```python
from build123d import *

# Parameters (mm, degrees)
SKETCH1_W                                           = 128
SKETCH1_H                                           = 28
BOSS_EXTRUDE1_DEPTH                                 = 45
SKETCH2_OUTSIDE_W                                   = 157.708
SKETCH2_OUTSIDE_H                                   = 74.708
CUT_EXTRUDE2_DEPTH                                  = 84.096329642
FILLET1_R                                           = 6
FILLET2_R                                           = 2
SKETCH3_W                                           = 16
SKETCH3_H                                           = 16
CUT_EXTRUDE3_DEPTH                                  = 29
FILLET3_R                                           = 2
CBORE_FOR_M8_HEX_SOCKET_HEAD_CAP_SCREW1_D           = 9
CBORE_FOR_M8_HEX_SOCKET_HEAD_CAP_SCREW1_DEPTH       = 15
CBORE_FOR_M8_HEX_SOCKET_HEAD_CAP_SCREW1_CBORE_D     = 15
CBORE_FOR_M8_HEX_SOCKET_HEAD_CAP_SCREW1_CBORE_DEPTH = 8.6
CBORE_FOR_M8_HEX_SOCKET_HEAD_CAP_SCREW1_TIP         = 2.703872786


with BuildPart() as part:
    # Sketch1 → Boss-Extrude1 (new body)
    with BuildSketch(Plane.XY):
        Rectangle(SKETCH1_W, SKETCH1_H)
    extrude(amount=BOSS_EXTRUDE1_DEPTH)

    # Sketch2 outside → Cut-Extrude2 (cut, through all)
    with BuildSketch(Plane.XZ.offset(14)):
        with Locations((0, 22.5)):
            Rectangle(SKETCH2_OUTSIDE_W, SKETCH2_OUTSIDE_H)
        Polygon((-47, 0), (-47, 38), (47, 38), (47, 0), (64, 0), (64, 16), (51, 45), (-51, 45), (-64, 16), (-64, 0), align=None, mode=Mode.SUBTRACT)
    extrude(amount=-CUT_EXTRUDE2_DEPTH, mode=Mode.SUBTRACT)

    # Fillet1
    fillet1_edges = [part.edges().sort_by_distance(p)[0] for p in [
        (-64, 0, 16),
        (-51, 0, 45),
        (51, 0, 45),
        (64, 0, 16),
    ]]
    fillet(fillet1_edges, radius=FILLET1_R)

    # Fillet2
    fillet2_edges = [part.edges().sort_by_distance(p)[0] for p in [
        (-47, 14, 19),
        (0, 14, 38),
        (47, -14, 19),
        (47, 14, 19),
        (47, 0, 38),
        (0, -14, 38),
        (-47, 0, 38),
        (-47, -14, 19),
        (0, -14, 45),
        (0, 14, 45),
        (-58.032245896, -14, 29.312682233),
        (-64, -14, 7.358346808),
        (64, -14, 7.358346808),
        (58.032245896, -14, 29.312682233),
        (63.867296468, -14, 15.971616785),
        (50.375820334, -14, 44.036169802),
        (-63.867296468, -14, 15.971616785),
        (-50.375820334, -14, 44.036169802),
        (-58.032245896, 14, 29.312682233),
        (58.032245896, 14, 29.312682233),
        (64, 14, 7.358346808),
        (-64, 14, 7.358346808),
        (63.867296468, 14, 15.971616785),
        (50.375820334, 14, 44.036169802),
        (-63.867296468, 14, 15.971616785),
        (-50.375820334, 14, 44.036169802),
    ]]
    fillet(fillet2_edges, radius=FILLET2_R)

    # Sketch3 → Cut-Extrude3 (cut)
    with BuildSketch(Plane.XY.offset(45)):
        with Locations((-56, 0)):
            Rectangle(SKETCH3_W, SKETCH3_H)
        with Locations((56, 0)):
            Rectangle(SKETCH3_W, SKETCH3_H)
    extrude(amount=-CUT_EXTRUDE3_DEPTH, mode=Mode.SUBTRACT)

    # Fillet3
    # the kernel refuses this fillet: 2 mm, written as the material it takes off along each edge
    with BuildSketch(Plane(origin=(63.861153873, -8, 16), x_dir=(0.06925637128898768, 0, -0.9975988948650063), z_dir=(0, 1, 0))) as fillet3_piece_1:
        with BuildLine():
            CenterArc((1.866301026, 1.99519779), FILLET3_R, 183.971276773, 90)
            Line((-0.128896764, 1.856685047), (-0.328416543, 1.842833773))
            Line((-0.328416543, 1.842833773), (-0.199519779, -0.013851274))
            Line((-0.199519779, -0.013851274), (-0.029143426, -0.197865259))
            ThreePointArc((-0.029143426, -0.197865259), (1.303692283, -0.249155378), (2.018665043, -0.199519779))
            Line((2.018665043, -0.199519779), (2.004813769, 0))
        make_face()
    extrude(amount=16, mode=Mode.SUBTRACT)
    with BuildSketch(Plane(origin=(48, -8, 44.934279824), x_dir=(-0.999460544146637, 0, 0.032842361274859504), z_dir=(0, 1, 0))) as fillet3_piece_2:
        with BuildLine():
            CenterArc((1.935394771, -1.998921088), FILLET3_R, 88.117932867, 90)
            Line((-0.063526317, -1.933236366), (-0.263418426, -1.926667893))
            Line((-0.263418426, -1.926667893), (-0.199892109, 0.006568472))
            Line((-0.199892109, 0.006568472), (-0.02300822, 0.198672147))
            ThreePointArc((-0.02300822, 0.198672147), (0.893869228, 0.236490976), (2.007647966, 0.199892109))
            Line((2.007647966, 0.199892109), (2.001079494, 0))
        make_face()
    extrude(amount=16, mode=Mode.SUBTRACT)
    with BuildSketch(Plane(origin=(-63.861153873, -8, 16), x_dir=(-0.06925637128898415, 0, -0.9975988948650065), z_dir=(0, 1, 0))) as fillet3_piece_3:
        with BuildLine():
            CenterArc((1.866301026, -1.99519779), FILLET3_R, 86.028723227, 90)
            Line((-0.128896764, -1.856685047), (-0.328416543, -1.842833773))
            Line((-0.328416543, -1.842833773), (-0.199519779, 0.013851274))
            Line((-0.199519779, 0.013851274), (-0.029143426, 0.197865259))
            ThreePointArc((-0.029143426, 0.197865259), (1.303692283, 0.249155378), (2.018665043, 0.199519779))
            Line((2.018665043, 0.199519779), (2.004813769, 0))
        make_face()
    extrude(amount=16, mode=Mode.SUBTRACT)
    with BuildSketch(Plane(origin=(-48, -8, 44.934279824), x_dir=(0.999460544146637, 0, 0.032842361274859504), z_dir=(0, 1, 0))) as fillet3_piece_4:
        with BuildLine():
            CenterArc((1.935394771, 1.998921088), FILLET3_R, 181.882067133, 90)
            Line((-0.063526317, 1.933236366), (-0.263418426, 1.926667893))
            Line((-0.263418426, 1.926667893), (-0.199892109, -0.006568472))
            Line((-0.199892109, -0.006568472), (-0.02300822, -0.198672147))
            ThreePointArc((-0.02300822, -0.198672147), (0.893869228, -0.236490976), (2.007647966, -0.199892109))
            Line((2.007647966, -0.199892109), (2.001079494, 0))
        make_face()
    extrude(amount=16, mode=Mode.SUBTRACT)

    # CBORE for M8 Hex Socket Head Cap Screw1
    with Locations(Plane.XY.offset(16)):
        with Locations((-56, 0), (56, 0)):
            CounterBoreHole(CBORE_FOR_M8_HEX_SOCKET_HEAD_CAP_SCREW1_D / 2, CBORE_FOR_M8_HEX_SOCKET_HEAD_CAP_SCREW1_CBORE_D / 2, CBORE_FOR_M8_HEX_SOCKET_HEAD_CAP_SCREW1_CBORE_DEPTH, depth=CBORE_FOR_M8_HEX_SOCKET_HEAD_CAP_SCREW1_DEPTH)
            with Locations((0, 0, -(CBORE_FOR_M8_HEX_SOCKET_HEAD_CAP_SCREW1_DEPTH + CBORE_FOR_M8_HEX_SOCKET_HEAD_CAP_SCREW1_TIP / 2))):  # 118° drill point
                Cone(0, CBORE_FOR_M8_HEX_SOCKET_HEAD_CAP_SCREW1_D / 2, CBORE_FOR_M8_HEX_SOCKET_HEAD_CAP_SCREW1_TIP, mode=Mode.SUBTRACT)


solid = part.part
```
Geometry: final body of the model. Coordinates: model frame, mm. A direction names the side the tool comes from. Round coordinates to 2 decimals unless told otherwise and drop trailing zeros. Write each loop counter-clockwise with the first axis right and the second up, starting at its lowest first coordinate (ties: lowest second). Pieces come first, ordered by that corner, then holes. Notation, with made-up numbers: M -5.75,57.25 L -1.75,57.25 A25 ccw -1.75,83.25 Z; hole C -4,-0.5 d6. An arc over 180 degrees is marked long. Answer in a Markdown table with one row per item. Add a question column.
(1) Cut plane C-C, the plane y = 10.5. Return the cut outline in (x, z), then the cut area to 3 significant figures.
(2) Cut plane B-B, the plane x = 10.5. Return the cut outline in (y, z), then the cut area to 3 significant figures.
(3) Draft query along X for faces 6 (the face through (63.87, -9.97, 15.95)), 7 (the face through (-48.846, 2.253, 11.76)), 8 (the face through (55, 3, 0)). Return one class per face: pulls with the +X half, pulls with the -X half, needs draft (parallel to the pull), parting line crosses it, or undercut.
(4) Reachability of faces 1 (the face through (50.416, -9.972, 44.01)), 2 (the face through (-50.416, -9.972, 44.01)), 3 (the face through (-60.292, 1.352, 4.155)), 4 (the face through (-48, 0, 30)), 5 (the face through (53, 8, 26)) from +Z, -Z, +X, -X, +Y, -Y: full face, straight path, thin tool, end or side. Return the list, or none.
(5) Cut plane A-A, the plane z = 9. Return the cut outline in (x, y), then the cut area to 3 significant figures.
(6) Cut plane D-D, the plane y = 0. Give the number of separate pieces and of enclosed holes in the cut face, then the cut area to 3 significant figures.
(7) Ray query, L1, parallel to X at y = 0, z = 13; L2, parallel to X at y = 0, z = 3; L3, parallel to X at y = 4.25, z = 24.5. Return the intervals inside material, ascending.
(8) Contact query for flat-ended pins moving along their axis: pin 1 (10 mm diameter, centred on y = -4.5, z = 31.5, fed in from -X); pin 2 (7 mm diameter, centred on x = 55.5, y = 3.5, fed in from +Z); pin 3 (6 mm diameter, centred on x = -32, z = 34.5, fed in from +Y); pin 4 (12 mm diameter, centred on x = 16, y = 6.5, fed in from -Z). Output: stop coordinate, or through.
Established:
| question | item | result |
|---|---|---|
| 1 | outline | M -64,0 L -47,0 L -47,36 A2 cw -45,38 L 45,38 A2 cw 47,36 L 47,0 L 64,0 L 64,14.72 A6 ccw 63.48,17.17 L 52.59,41.45 A6 ccw 47.11,45 L -47.11,45 A6 ccw -52.59,41.45 L -63.48,17.17 A6 ccw -64,14.72 Z |
| 1 | area | 1,810 mm² |
| 2 | outline | M -14,40 A2 ccw -12,38 L 12,38 A2 ccw 14,40 L 14,43 A2 ccw 12,45 L -12,45 A2 ccw -14,43 Z |
| 2 | area | 193 mm² |
| 3 | face 6 | pulls with the +X half |
| 3 | face 7 | undercut |
| 3 | face 8 | needs draft |
| 4 | face 1 | +Z, +X, +Y, -Y |
| 4 | face 2 | +Z, -X, +Y, -Y |
| 4 | face 3 | +Z |
| 4 | face 4 | +Z, -X |
| 4 | face 5 | +Z, +X |
| 5 | outline | M -64,-12 A2 ccw -62,-14 L -49,-14 A2 ccw -47,-12 L -47,12 A2 ccw -49,14 L -62,14 A2 ccw -64,12 Z; M 47,-12 A2 ccw 49,-14 L 62,-14 A2 ccw 64,-12 L 64,12 A2 ccw 62,14 L 49,14 A2 ccw 47,12 Z; hole C -56,0 d15; hole C 56,0 d15 |
| 5 | area | 592 mm² |
| 6 | separate pieces | 3 |
| 6 | enclosed holes | 0 |
| 6 | area | 871 mm² |
| 7 | L1 | -64 to -63.5, -48.5 to -47, 47 to 48.5, 63.5 to 64 |
| 7 | L2 | -64 to -60.5, -51.5 to -47, 47 to 51.5, 60.5 to 64 |
| 7 | L3 | -48 to -47, 47 to 48 |
| 8 | pin 1 | x = -58.65 |
| 8 | pin 2 | z = 7.4 |
| 8 | pin 3 | through |
| 8 | pin 4 | z = 38 |
